Can you work these out from the drawing? Everything is in mm from the part's minimum corner. Round coordinates to 2 decimals unless told otherwise and drop trailing zeros. Order: outer loops, then holes, each group sorted by start corner. A loop starts at its lowest first (then second) coordinate and runs counter-clockwise, first axis right, second up. Notation, with made-up numbers: (57.25, 67) -> (86.25, 67) arc R21 cw to (86.25, 85) -> close; hole circle Ø11 at (-25, 79). An arc over 180 degrees is marked (long way). One line per item, written item: value.
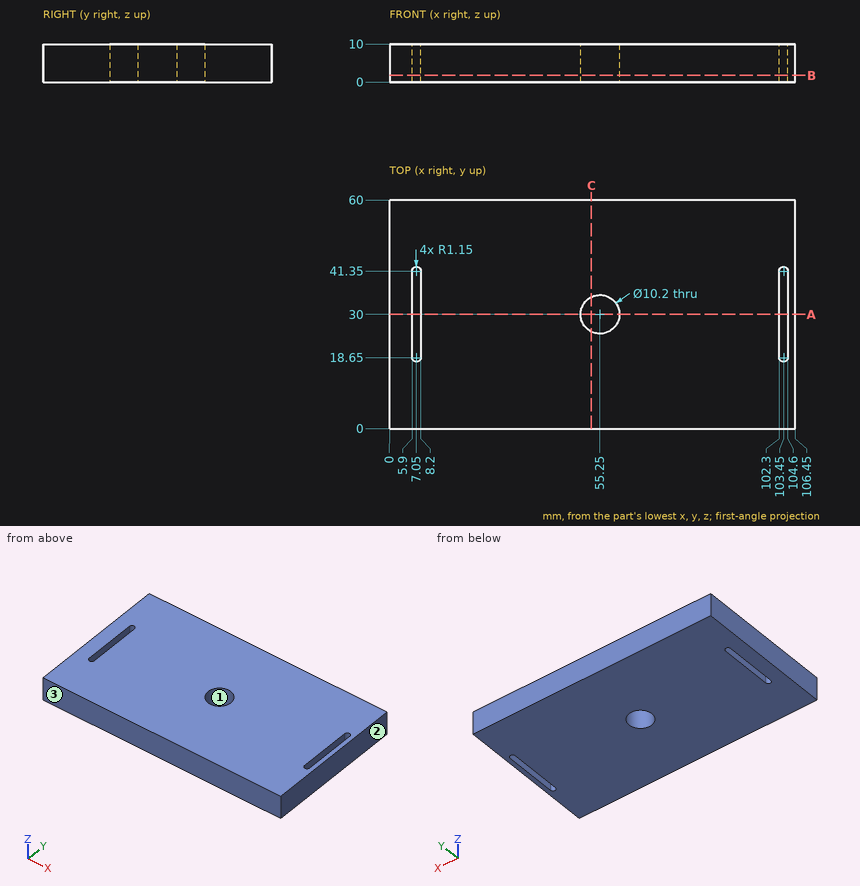
Q1. We'd pull the mould along Y, two halves only. Please class the marked faces 1, 2 and 3: released by +Y, released by -Y, zero draft, split by the parting line, or undercut.
Answers below:
face 1: undercut
face 2: zero draft
face 3: released by -Y
Q2. I want a section at A-A on y = 30. List the corners of the cut face in (x, z) for me.
Answers below:
outline: (0, 0) -> (5.9, 0) -> (5.9, 10) -> (0, 10) -> close; (8.2, 0) -> (50.15, 0) -> (50.15, 10) -> (8.2, 10) -> close; (60.35, 0) -> (102.3, 0) -> (102.3, 10) -> (60.35, 10) -> close; (104.6, 0) -> (106.45, 0) -> (106.45, 10) -> (104.6, 10) -> close
Q3. Please list where these lines run through material, in increasing order: line 1 along X through (y, z) = (35.5, 0.5); line 2 along Y through (x, z) = (51.5, 7.75) (1 decimal).
Answers below:
line 1: 0 to 5.9, 8.2 to 102.3, 104.6 to 106.45
line 2: 0 to 26.5, 33.5 to 60
Q4. I want a section at C-C on x = 53. List the corners of the cut face in (y, z) for me.
Answers below:
outline: (0, 0) -> (25.42, 0) -> (25.42, 10) -> (0, 10) -> close; (34.58, 0) -> (60, 0) -> (60, 10) -> (34.58, 10) -> close
Q5. I want a section at B-B on z = 1.75. List the corners of the cut face in (x, y) for me.
Answers below:
outline: (0, 0) -> (106.45, 0) -> (106.45, 60) -> (0, 60) -> close; hole (5.9, 18.65) arc R1.15 ccw to (8.2, 18.65) -> (8.2, 41.35) arc R1.15 ccw to (5.9, 41.35) -> close; hole circle Ø10.2 at (55.25, 30); hole (102.3, 18.65) arc R1.15 ccw to (104.6, 18.65) -> (104.6, 41.35) arc R1.15 ccw to (102.3, 41.35) -> close
